Input: part model. Units: mm. Frame: model coordinates. Coordinates: 2 decimals unless noted, no trailing zeros. Loops run counter-clockwise (first coordinate to the right, second up) from the corner with the lowest first, then second, coordinate; pieces in that order, holes last.
(1) Section D-D, the plane x = 18.5. Return loops of the section in (y, z).
(2) Section B-B, the plane x = -7. Return loops of the section in (y, z), then the cut area to 3 significant figures.
(3) Contact query for flat-ended pins moving along their axis: P1, Ø1, axis at y = 1, z = -317.5, coming from the -X side; P2, Ø0.7, axis at y = 1.5, z = -305.5, coming from the +X side; P3, Ø1, axis at x = -4, y = 1, coming from the -Z side. Output: stop coordinate, or through.
(4) Line query: L1, parallel to X at y = 1.25, z = -335; L2, parallel to Z at x = -7, y = 1.3; L3, parallel to X at y = 1.2, z = -332.5. Output: solid intervals per line, ascending.
(5) Section A-A, the plane z = -317.15. Return loops of the section in (x, y), then the cut area to 3 significant figures.
(6) Section C-C, the plane y = 0.95. Give the number of separate pieces and of enclosed holes in the cut face, then the cut area to 3 significant figures.
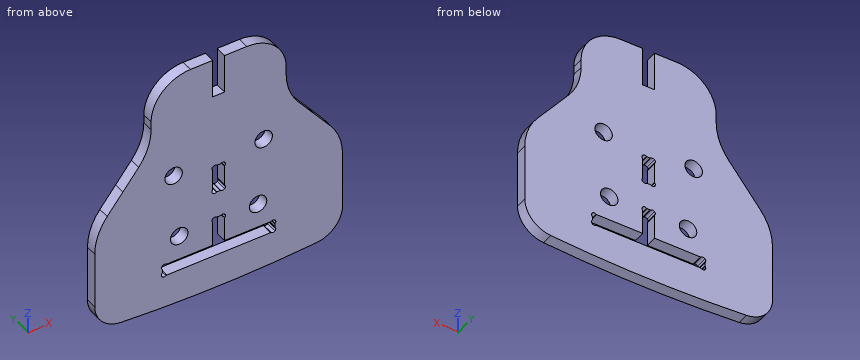
```python
from build123d import *

# Parameters (mm, degrees)
EXTRUDE_1_DEPTH     = 2
SKETCH_2_W          = 1.05
SKETCH_2_H          = 5.1
CUT_EXTRUDE_1_DEPTH = 343.513123836
CUT_EXTRUDE_2_DEPTH = 343.513123836
FILLET_1_R          = 0.2
SKETCH_4_R          = 1.55
CUT_EXTRUDE_3_DEPTH = 343.513123836
FILLET_2_R          = 5
EXTRUDE_START       = -2
EXTRUDE_2_DEPTH     = 2
CUT_EXTRUDE_START   = -10
CUT_EXTRUDE_5_DEPTH = 10
SKETCH_6_W          = 2.1
SKETCH_6_H          = 7
CUT_EXTRUDE_4_DEPTH = 2
FILLET_8_R          = 7
FILLET_5_R          = 10
FILLET_6_R          = 10


with BuildPart() as part:
    # 草图1 → 凸台-拉伸1 (new body)
    with BuildSketch(Plane(origin=(0, 0, 0), x_dir=(1, 0, 0), z_dir=(0, 1, 0))):
        with BuildLine():
            Line((-22, 322.5), (-17, 320.227272727))
            Line((-17, 320.227272727), (-17, 312.037257391))
            ThreePointArc((-17, 312.037257391), (0, 312.5), (17, 312.037257391))
            Line((17, 312.037257391), (17, 320.227272727))
            Line((17, 320.227272727), (22, 322.5))
            Line((22, 322.5), (22, 340.767946523))
            ThreePointArc((22, 340.767946523), (0, 341.8), (-22, 340.767946523))
            Line((-22, 340.767946523), (-22, 322.5))
        make_face()
    extrude(amount=EXTRUDE_1_DEPTH)

    # 草图2 → 切除-拉伸1 (cut, through all)
    with BuildSketch(Plane(origin=(0, 2, 0), x_dir=(1, 0, 0), z_dir=(0, 1, 0))):
        Polygon((0, 335.65), (0, 328.45), (1.05, 328.45), (1.05, 333.55), (10, 333.55), (10, 335.65), align=None)
        Polygon((-1.05, 328.45), (0, 328.45), (0, 335.65), (-10, 335.65), (-10, 333.55), (-1.05, 333.55), align=None)
        with Locations((0.525, 321.05)):
            Rectangle(SKETCH_2_W, SKETCH_2_H)
        with Locations((-0.525, 321.05)):
            Rectangle(SKETCH_2_W, SKETCH_2_H)
    extrude(amount=-CUT_EXTRUDE_1_DEPTH, mode=Mode.SUBTRACT)

    # 草图3 → 切除-拉伸2 (cut, through all)
    with BuildSketch(Plane(origin=(0, 2, 0), x_dir=(1, 0, 0), z_dir=(0, 1, 0))):
        with BuildLine():
            Line((10, 335.65), (10, 334.942893219))
            ThreePointArc((10, 334.942893219), (10.108386376, 335.105104893), (10.146446609, 335.296446609))
            ThreePointArc((10.146446609, 335.296446609), (10.108386376, 335.487788326), (10, 335.65))
        make_face()
        with BuildLine():
            ThreePointArc((10, 335.65), (9.646446609, 335.796446609), (9.292893219, 335.65))
            Line((9.292893219, 335.65), (10, 335.65))
        make_face()
        with BuildLine():
            ThreePointArc((10.146446609, 333.903553391), (10.108386376, 334.094895107), (10, 334.257106781))
            Line((10, 334.257106781), (10, 333.55))
            ThreePointArc((10, 333.55), (10.108386376, 333.712211674), (10.146446609, 333.903553391))
        make_face()
        with BuildLine():
            Line((10, 333.55), (9.292893219, 333.55))
            ThreePointArc((9.292893219, 333.55), (9.646446609, 333.403553391), (10, 333.55))
        make_face()
        with BuildLine():
            ThreePointArc((1.196446609, 328.803553391), (1.158386376, 328.994895107), (1.05, 329.157106781))
            Line((1.05, 329.157106781), (1.05, 328.45))
            ThreePointArc((1.05, 328.45), (1.158386376, 328.612211674), (1.196446609, 328.803553391))
        make_face()
        with BuildLine():
            Line((1.05, 328.45), (0.342893219, 328.45))
            ThreePointArc((0.342893219, 328.45), (0.696446609, 328.303553391), (1.05, 328.45))
        make_face()
        with BuildLine():
            ThreePointArc((1.196446609, 323.246446609), (1.158386376, 323.437788326), (1.05, 323.6))
            Line((1.05, 323.6), (1.05, 322.892893219))
            ThreePointArc((1.05, 322.892893219), (1.158386376, 323.055104893), (1.196446609, 323.246446609))
        make_face()
        with BuildLine():
            ThreePointArc((1.05, 323.6), (0.696446609, 323.746446609), (0.342893219, 323.6))
            Line((0.342893219, 323.6), (1.05, 323.6))
        make_face()
        with BuildLine():
            ThreePointArc((1.196446609, 318.853553391), (1.158386376, 319.044895107), (1.05, 319.207106781))
            Line((1.05, 319.207106781), (1.05, 318.5))
            ThreePointArc((1.05, 318.5), (1.158386376, 318.662211674), (1.196446609, 318.853553391))
        make_face()
        with BuildLine():
            Line((1.05, 318.5), (0.342893219, 318.5))
            ThreePointArc((0.342893219, 318.5), (0.696446609, 318.353553391), (1.05, 318.5))
        make_face()
    cut_extrude_2 = extrude(amount=-CUT_EXTRUDE_2_DEPTH, mode=Mode.SUBTRACT)

    # 镜向1: 切除-拉伸2 across plane
    add(cut_extrude_2.mirror(Plane(origin=(0, 0, 0), x_dir=(0, 0, 1), z_dir=(1, 0, 0))), mode=Mode.SUBTRACT)

    # 圆角1
    fillet_1_edges = [part.edges().sort_by_distance(p)[0] for p in [
        (1.05, 1, -329.157106781),
        (0.342893219, 1, -323.6),
        (1.05, 1, -319.207106781),
        (9.292893219, 1, -335.65),
        (10, 1, -334.257106781),
        (0.342893219, 1, -328.45),
        (1.05, 1, -322.892893219),
        (0.342893219, 1, -318.5),
        (-10, 1, -334.942893219),
        (-9.292893219, 1, -333.55),
        (-1.05, 1, -329.157106781),
        (-0.342893219, 1, -323.6),
        (-1.05, 1, -319.207106781),
        (-9.292893219, 1, -335.65),
        (-10, 1, -334.257106781),
        (-0.342893219, 1, -328.45),
        (-1.05, 1, -322.892893219),
        (-0.342893219, 1, -318.5),
        (10, 1, -334.942893219),
        (9.292893219, 1, -333.55),
    ]]
    fillet(fillet_1_edges, radius=FILLET_1_R)

    # 草图4 → 切除-拉伸3 (cut, through all)
    with BuildSketch(Plane(origin=(0, 2, 0), x_dir=(1, 0, 0), z_dir=(0, 1, 0))):
        with Locations(Location((7, 329.15, 0), (0, 0, 270))):
            Circle(SKETCH_4_R)
        with Locations(Location((8, 317.15, 0), (0, 0, 270))):
            Circle(SKETCH_4_R)
    cut_extrude_3 = extrude(amount=-CUT_EXTRUDE_3_DEPTH, mode=Mode.SUBTRACT)

    # 镜向2: 切除-拉伸3 across plane
    add(cut_extrude_3.mirror(Plane(origin=(0, 0, 0), x_dir=(0, 0, 1), z_dir=(1, 0, 0))), mode=Mode.SUBTRACT)

    # 圆角2
    fillet_2_edges = [part.edges().sort_by_distance(p)[0] for p in [
        (-22, 1, -340.767946523),
        (22, 1, -340.767946523),
    ]]
    fillet(fillet_2_edges, radius=FILLET_2_R)

    # 草图5 → 凸台-拉伸2 (add)
    with BuildSketch(Plane(origin=(0, 2, 0), x_dir=(1, 0, 0), z_dir=(0, 1, 0)).offset(EXTRUDE_START)):
        with BuildLine():
            Line((-13.733814581, 312.198065877), (-12, 310.037257391))
            Line((-12, 310.037257391), (-12, 298.037257391))
            Line((-12, 298.037257391), (12, 298.037257391))
            Line((12, 298.037257391), (12, 310.037257391))
            Line((12, 310.037257391), (13.733814581, 312.198065877))
            ThreePointArc((13.733814581, 312.198065877), (0, 312.5), (-13.733814581, 312.198065877))
        make_face()
        Polygon((-22, 322.5), (-17, 316.268628695), (-17, 320.227272727), align=None)
        Polygon((17, 316.268628695), (22, 322.5), (17, 320.227272727), align=None)
    extrude(amount=EXTRUDE_2_DEPTH)

    # 草图5<3> → 切除-拉伸5 (cut)
    with BuildSketch(Plane(origin=(0, 2, 0), x_dir=(1, 0, 0), z_dir=(0, 1, 0)).offset(CUT_EXTRUDE_START)):
        with BuildLine():
            Line((-17, 310.037257391), (-17, 312.037257391))
            ThreePointArc((-17, 312.037257391), (-15.367117639, 312.121934019), (-13.733814581, 312.198065877))
            Line((-13.733814581, 312.198065877), (-22, 322.5))
            Line((-22, 322.5), (-22, 310.037257391))
            Line((-22, 310.037257391), (-17, 310.037257391))
        make_face()
        with BuildLine():
            ThreePointArc((-13.733814581, 312.198065877), (-15.367117639, 312.121934019), (-17, 312.037257391))
            Line((-17, 312.037257391), (-17, 310.037257391))
            Line((-17, 310.037257391), (-12, 310.037257391))
            Line((-12, 310.037257391), (-13.733814581, 312.198065877))
        make_face()
        with BuildLine():
            Line((22, 322.5), (13.733814581, 312.198065877))
            ThreePointArc((13.733814581, 312.198065877), (15.367117639, 312.121934019), (17, 312.037257391))
            Line((17, 312.037257391), (17, 310.037257391))
            Line((17, 310.037257391), (22, 310.037257391))
            Line((22, 310.037257391), (22, 322.5))
        make_face()
        with BuildLine():
            Line((13.733814581, 312.198065877), (12, 310.037257391))
            Line((12, 310.037257391), (17, 310.037257391))
            Line((17, 310.037257391), (17, 312.037257391))
            ThreePointArc((17, 312.037257391), (15.367117639, 312.121934019), (13.733814581, 312.198065877))
        make_face()
    extrude(amount=CUT_EXTRUDE_5_DEPTH, mode=Mode.SUBTRACT)

    # 草图6 → 切除-拉伸4 (cut)
    with BuildSketch(Plane(origin=(0, 2, 0), x_dir=(1, 0, 0), z_dir=(0, 1, 0))):
        with Locations((0, 301.537257391)):
            Rectangle(SKETCH_6_W, SKETCH_6_H)
    extrude(amount=-CUT_EXTRUDE_4_DEPTH, mode=Mode.SUBTRACT)

    # 圆角8
    fillet_8_edges = [part.edges().sort_by_distance(p)[0] for p in [
        (12, 1, -298.037257391),
        (-12, 1, -298.037257391),
    ]]
    fillet(fillet_8_edges, radius=FILLET_8_R)

    # 圆角5
    fillet_5_edges = [part.edges().sort_by_distance(p)[0] for p in [
        (22, 1, -322.5),
        (-22, 1, -322.5),
    ]]
    fillet(fillet_5_edges, radius=FILLET_5_R)

    # 圆角6
    fillet_6_edges = [part.edges().sort_by_distance(p)[0] for p in [
        (12, 1, -310.037257391),
        (-12, 1, -310.037257391),
    ]]
    fillet(fillet_6_edges, radius=FILLET_6_R)


solid = part.part
```
Report:
1. outline: (0, -340.94) - (2, -340.94) - (2, -318.14) - (0, -318.14) - close
2. outline: (0, -341.7) - (2, -341.7) - (2, -335.65) - (0, -335.65) - close; (0, -333.55) - (2, -333.55) - (2, -330.7) - (0, -330.7) - close; (0, -327.6) - (2, -327.6) - (2, -318.33) - (0, -318.33) - close; (0, -315.97) - (2, -315.97) - (2, -298.33) - (0, -298.33) - close
2. area: 71.6 mm2
3. P1: stops at x = -18.39
3. P2: stops at x = 12
3. P3: stops at z = -341.77
4. L1: x = -22 to -10.05, 10.05 to 22
4. L2: z = -341.7 to -335.65, -333.55 to -330.7, -327.6 to -318.33, -315.97 to -298.33
4. L3: x = -22 to -1.05, 1.05 to 22
5. outline: (-17.71, 0) - (-9.55, 0) - (-9.55, 2) - (-17.71, 2) - close; (-6.45, 0) - (6.45, 0) - (6.45, 2) - (-6.45, 2) - close; (9.55, 0) - (17.71, 0) - (17.71, 2) - (9.55, 2) - close
5. area: 58.4 mm2
6. separate pieces: 1
6. enclosed holes: 6
6. area: 1,410 mm2
